Geometry check sheet. Reference: the model listing, model coordinates, mm. A direction names the side the tool comes from. Round coordinates to 2 decimals unless told otherwise and drop trailing zeros. Order: outer loops, then holes, each group sorted by start corner. A loop starts at its lowest first (then second) coordinate and runs counter-clockwise, first axis right, second up.
```python
from build123d import *

# Parameters (mm, degrees)
F6_W     = 127
F6_H     = 69.85
F0_DEPTH = 6.35
F1_R     = 6.35
F2_DEPTH = 127
F7_R     = 3.81
F8_DEPTH = 127
F3_R     = 2.54
F4_DEPTH = 5.08
F9_R     = 2.54
F5_DEPTH = 5.08


with BuildPart() as f0:
    # F6 (on Front) → F0 (new body)
    with BuildSketch(Plane.XZ):
        with Locations((-32.109398, 34.925)):
            Rectangle(F6_W, F6_H)
    extrude(amount=F0_DEPTH)

    # F1 (on face) → F2 (join)
    with BuildSketch(Plane.YZ.offset(31.390602)):
        with Locations((0, 54.61)):
            Circle(F1_R)
        with Locations((0, 15.24)):
            Circle(F1_R)
    extrude(amount=-F2_DEPTH)

    # F7 (on face) → F8 (cut)
    with BuildSketch(Plane.YZ.offset(31.390602)):
        with Locations((0, 54.61)):
            Circle(F7_R)
        with Locations((0, 15.24)):
            Circle(F7_R)
    extrude(amount=-F8_DEPTH, mode=Mode.SUBTRACT)

    # F3 (on face) → F4 (join)
    with BuildSketch(Plane.XZ.offset(6.35)):
        with Locations((-51.159398, 6.35)):
            Circle(F3_R)
        with Locations((-51.159398, 22.86)):
            Circle(F3_R)
        with Locations((18.690602, 6.35)):
            Circle(F3_R)
        with Locations((18.690602, 22.86)):
            Circle(F3_R)
    extrude(amount=F4_DEPTH)

    # F9 (on face) → F5 (join)
    with BuildSketch(Plane.XZ.offset(6.35)):
        with Locations((-42.269398, 43.18)):
            Circle(F9_R)
        with Locations((-42.269398, 63.5)):
            Circle(F9_R)
        with Locations((18.690602, 43.18)):
            Circle(F9_R)
        with Locations((18.690602, 63.5)):
            Circle(F9_R)
    extrude(amount=F5_DEPTH)


solid = f0.part
```
(1) Sectioned sample at B-B, the plane x = -67. Record the cut outline in (y, z).
Returned:
outline: (-6.35, 0) - (0, 0) - (0, 8.89) arc R6.35 ccw to (0, 21.59) - (0, 48.26) arc R6.35 ccw to (0, 60.96) - (0, 69.85) - (-6.35, 69.85) - close; hole circle Ø7.62 at (0, 15.24); hole circle Ø7.62 at (0, 54.61)
(2) Sectioned sample at C-C, the plane z = 43.18. Record the cut outline in (x, y), and give its area (3 significant figures).
Returned:
outline: (-95.61, -6.35) - (-44.81, -6.35) - (-44.81, -11.43) - (-39.73, -11.43) - (-39.73, -6.35) - (16.15, -6.35) - (16.15, -11.43) - (21.23, -11.43) - (21.23, -6.35) - (31.39, -6.35) - (31.39, 0) - (-95.61, 0) - close
area: 858 mm2
(3) Sectioned sample at D-D, the plane z = 52. Record the cut outline in (x, y), and give its area (3 significant figures).
Returned:
outline: (-95.61, -6.35) - (31.39, -6.35) - (31.39, -2.78) - (-95.61, -2.78) - close; (-95.61, 2.78) - (31.39, 2.78) - (31.39, 5.79) - (-95.61, 5.79) - close
area: 837 mm2
(4) Draft check along Z on faces 1 (the cylindrical face through (-53.175, -8.854, 21.314)), 2 (the flat face through (-33, -3, 69.85)), 3 (the flat face through (19, -11.43, 43)). Enter one of: released by +Z, released by -Z, zero draft, split by the parting line, or undercut.
Returned:
face 1: undercut
face 2: released by +Z
face 3: zero draft
(5) Set-up check for faces 4 (the flat face through (-33, 0, 65)), 5 (the flat face through (-33, 0, 5)), 6 (the cylindrical face through (-53.697, -8.854, 6.462)): record each of +Z, -Z, +X, -X, +Y, -Y from which the full face is reachable in a straight line by a thin tool's end or side.
Returned:
face 4: +Z, +X, -X, +Y
face 5: -Z, +X, -X, +Y
face 6: -Y
(6) Depth check by flat-ended pin: P1, Ø1.5, axis at y = 3, z = 8.5, coming from the -X side; P2, Ø4, axis at x = -60.5, z = 19, coming from the -Y side; P3, Ø7, axis at x = -49, z = 2.5, coming from the +Y side. Enter the tip coordinate at first touch or a pass-through.
Returned:
P1: passes through
P2: stops at y = -6.35
P3: stops at y = 0
(7) Material ranges on line 1 (Z direction, x = -38, y = 1); line 2 (Y direction, x = -24, z = 15); line 3 (Y direction, x = -76, z = 5.5), recorded low to high.
Returned:
line 1: z = 8.97 to 11.56, 18.92 to 21.51, 48.34 to 50.93, 58.29 to 60.88
line 2: y = -6.35 to -3.8, 3.8 to 6.35
line 3: y = -6.35 to 0
(8) Sectioned sample at A-A, the plane z = 15.24. Record the cut outline in (x, y), and give its area (3 significant figures).
Returned:
outline: (-95.61, -6.35) - (31.39, -6.35) - (31.39, -3.81) - (-95.61, -3.81) - close; (-95.61, 3.81) - (31.39, 3.81) - (31.39, 6.35) - (-95.61, 6.35) - close
area: 645 mm2
